Study the drawing (mm; zero at the part's minimum x, y, z) and answer. Round coordinates to 2 decimals unless told otherwise and drop trailing zeros. Write each loop counter-clockwise with the first axis right and the second up, starting at its lowest first coordinate (ties: lowest second). Pieces come first, ordered by that corner, then holes.
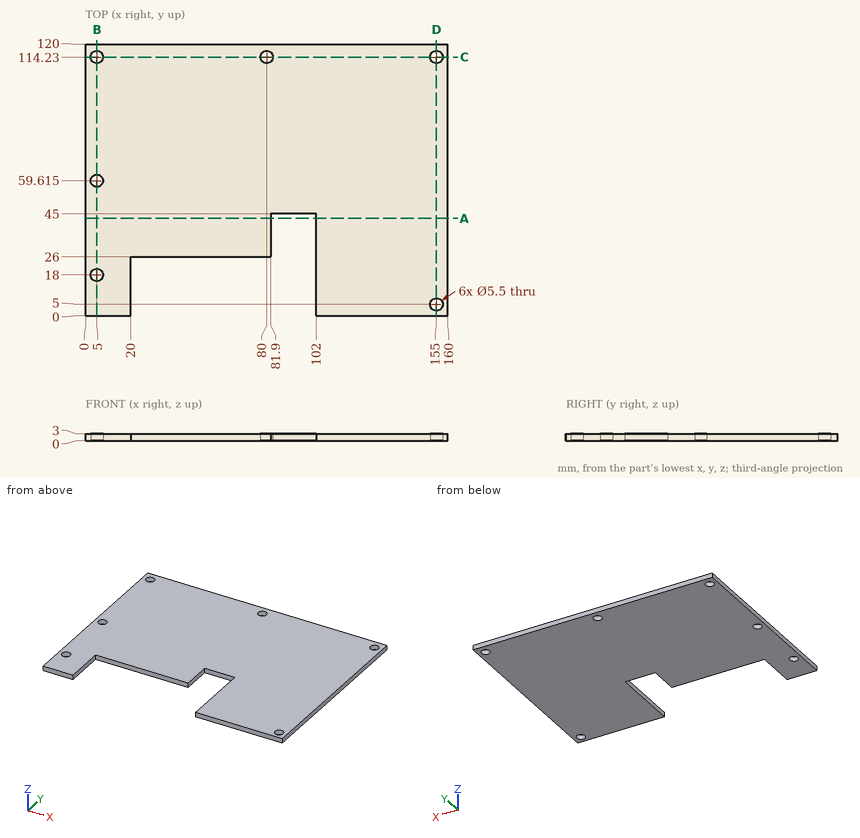
1. Section B-B on x = 5 is taken. Determine the outline of the cut face in (y, z) (3 decimals).
Geometry says:
outline: (0, 0) - (15.25, 0) - (15.25, 3) - (0, 3) - close; (20.75, 0) - (56.865, 0) - (56.865, 3) - (20.75, 3) - close; (62.365, 0) - (111.48, 0) - (111.48, 3) - (62.365, 3) - close; (116.98, 0) - (120, 0) - (120, 3) - (116.98, 3) - close
2. Section C-C on y = 114.23 is taken. Determine the outline of the cut face in (x, z).
Geometry says:
outline: (0, 0) - (2.25, 0) - (2.25, 3) - (0, 3) - close; (7.75, 0) - (77.25, 0) - (77.25, 3) - (7.75, 3) - close; (82.75, 0) - (152.25, 0) - (152.25, 3) - (82.75, 3) - close; (157.75, 0) - (160, 0) - (160, 3) - (157.75, 3) - close
3. Section D-D on x = 155 is taken. Determine the outline of the cut face in (y, z).
Geometry says:
outline: (0, 0) - (2.25, 0) - (2.25, 3) - (0, 3) - close; (7.75, 0) - (111.48, 0) - (111.48, 3) - (7.75, 3) - close; (116.98, 0) - (120, 0) - (120, 3) - (116.98, 3) - close
4. Section A-A on y = 43 is taken. Determine the outline of the cut face in (x, z), plus the area to 3 significant figures.
Geometry says:
outline: (0, 0) - (81.9, 0) - (81.9, 3) - (0, 3) - close; (102, 0) - (160, 0) - (160, 3) - (102, 3) - close
area: 420 mm2
5. Straight lines are drawn through the part: line 1 along Y through (x, z) = (5, 1.3) (3 decimals); line 2 along Y through (x, z) = (155, 2.15); line 3 along X through (y, z) = (15, 0.85). For each, find the intervals that lie inside material, in ascending order.
Geometry says:
line 1: y = 0 to 15.25, 20.75 to 56.865, 62.365 to 111.48, 116.98 to 120
line 2: y = 0 to 2.25, 7.75 to 111.48, 116.98 to 120
line 3: x = 0 to 20, 102 to 160
6. Given pin 1 (3.5 mm diameter, centred on x = 155, y = 5, fed in from +Z); pin 2 (1.5 mm diameter, centred on x = 40.5, z = 2, fed in from -Y); pin 3 (1.5 mm diameter, centred on x = 98.5, z = 1, fed in from -Y), each flat-ended and moving along its own axis, determine where each tip first touches the part or whether it passes through.
Geometry says:
pin 1: passes through
pin 2: stops at y = 26
pin 3: stops at y = 45
